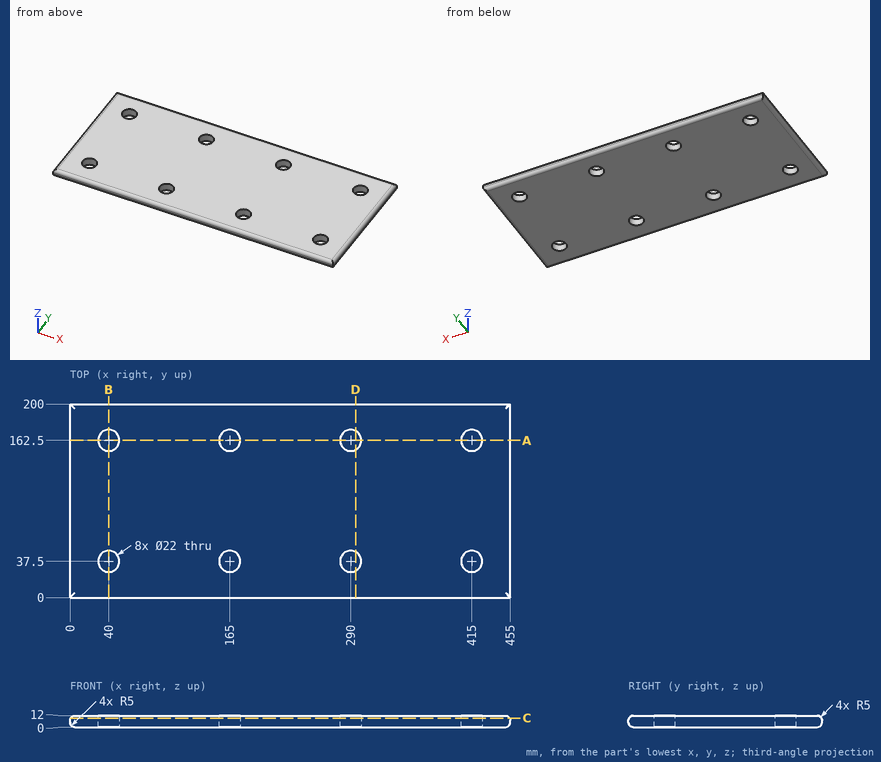
The figure shows three views and two pictorial views of one solid part (mm, origin at its lowest corner). Answer the questions. Round coordinates to 2 decimals unless told otherwise and drop trailing zeros. Write each loop counter-clockwise with the first axis right and the second up, starting at its lowest first coordinate (ties: lowest second). Pieces come first, ordered by that corner, then holes. Notation, with made-up numbers: M 26.25,44 L 67.25,44 A7 ccw 67.25,48 Z; hole C -18,23.5 d4. An arc over 180 degrees is marked long. Use a Markdown table: item, result.
1) The part is cut by section B-B (x = 40). Write down the section's boundary in (y, z).
Answers follow:
| item | result |
|---|---|
| outline | M 0,5 A5 ccw 5,0 L 26.5,0 L 26.5,12 L 5,12 A5 ccw 0,7 Z; M 48.5,0 L 151.5,0 L 151.5,12 L 48.5,12 Z; M 173.5,0 L 195,0 A5 ccw 200,5 L 200,7 A5 ccw 195,12 L 173.5,12 Z |
2) Straight lines are drawn through the part: line 1 along Y through (x, z) = (290, 7.5); line 2 along X through (y, z) = (31, 0.75); line 3 along Y through (x, z) = (40, 3.5). For each, find the intervals that lie inside material, in ascending order. Write a range as [from, to].
Answers follow:
| item | result |
|---|---|
| line 1 | y = [0.03, 26.5], [48.5, 151.5], [173.5, 199.97] |
| line 2 | x = [2.37, 31.13], [48.87, 156.13], [173.87, 281.13], [298.87, 406.13], [423.87, 452.63] |
| line 3 | y = [0.23, 26.5], [48.5, 151.5], [173.5, 199.77] |
3) The part is cut by section D-D (x = 295). Write down the section's boundary in (y, z).
Answers follow:
| item | result |
|---|---|
| outline | M 0,5 A5 ccw 5,0 L 27.7,0 L 27.7,12 L 5,12 A5 ccw 0,7 Z; M 47.3,0 L 152.7,0 L 152.7,12 L 47.3,12 Z; M 172.3,0 L 195,0 A5 ccw 200,5 L 200,7 A5 ccw 195,12 L 172.3,12 Z |
4) The part is cut by section C-C (z = 9.25). Give the number of separate pieces and of enclosed holes in the cut face, plus the area to 3 significant figures.
Answers follow:
| item | result |
|---|---|
| separate pieces | 1 |
| enclosed holes | 8 |
| area | 87,300 mm2 |
5) Flat-ended cylindrical pins translate along their axes: pin 1 (13 mm diameter, centred on x = 165, y = 37.5, fed in from +Z); pin 2 (1.5 mm diameter, centred on y = 94.5, z = 8.5, fed in from -X). Find the tip coordinate at first contact, or state that the pin passes through.
Answers follow:
| item | result |
|---|---|
| pin 1 | passes through |
| pin 2 | stops at x = 0.06 |
6) The part is cut by section A-A (y = 162.5). Write down the section's boundary in (x, z), plus the area to 3 significant figures.
Answers follow:
| item | result |
|---|---|
| outline | M 0,5 A5 ccw 5,0 L 29,0 L 29,12 L 5,12 A5 ccw 0,7 Z; M 51,0 L 154,0 L 154,12 L 51,12 Z; M 176,0 L 279,0 L 279,12 L 176,12 Z; M 301,0 L 404,0 L 404,12 L 301,12 Z; M 426,0 L 450,0 A5 ccw 455,5 L 455,7 A5 ccw 450,12 L 426,12 Z |
| area | 4,380 mm2 |
